Check sheet for the modelled part. Datum: model origin and axes. Units: mm. A direction names the side the tool comes from. Give positions to 0.01 mm unless a question says otherwise; leave off trailing zeros. Write each loop counter-clockwise with the first axis right and the second up, starting at its lowest first coordinate (ties: lowest second). Pieces come first, ordered by that corner, then holes. Notation, with made-up numbers: (-25.75, -9) -> (31.25, -9) arc R15 cw to (31.25, 7) -> close; hole circle Ø3 at (40.5, 18.25). An arc over 180 degrees is marked (long way). Use a Markdown table: item, result. Add a question column.
1. Cross-section at B-B (z = -26.7). Enter the section's corners in (x, y).
2. Scan lines: probe 1 along X at (y, z) = (2.5, 40.5); probe 2 along X at (y, z) = (3.8, 16.25); probe 3 along Z at (x, y) = (-18, 7). Record each from-to range of solid material in increasing order. Write a range as [from, to].
3. Cross-section at C-C (z = 0). Enter the section's corners in (x, y), then the cut area to 3 significant figures.
4. Set-up check for faces 1 (the flat face through (-49.65, 5, -7)), 2 (the flat face through (10.75, 4, -39)), 3 (the flat face through (18, 5, 1)): record each of +Z, -Z, +X, -X, +Y, -Y from which the full face is reachable in a straight line by a thin tool's end or side.
5. Cross-section at A-A (x = -36.95). Enter the section's corners in (y, z), then the cut area to 3 significant figures.
6. Release check for a two-part mould opening along X. For faces 4 (the flat face through (-12.75, 3, 1)), 5 (the flat face through (-21.25, 7, 1)), 6 (the flat face through (-51, 7, 10)) record: released by +X, released by -X, zero draft, split by the parting line, or undercut.
7. Cross-section at D-D (x = 0). Count the separate pieces of the cut face and the enclosed holes in it, then the cut area to 3 significant figures.
8. Gauge pin test, flat ends, axial feed: P1, Ø4, axis at x = -14.5, z = 10.5, coming from the +Y side; P2, Ø4, axis at y = 8, z = 13, coming from the -X side; P3, Ø1.5, axis at x = -27, y = 7.5, coming from the -Z side. Record the tip position at first contact, or that the pin passes through.
from build123d import *

# Parameters (mm, degrees)
BOSS_EXTRUDE1_DEPTH            = 45
SKETCH3_R                      = 6.5
CUT_EXTRUDE1_DEPTH             = 50.199212392
SKETCH5_W                      = 5
SKETCH5_H                      = 10
BOSS_EXTRUDE2_DEPTH            = 45
BOSS_EXTRUDE2_DEPTH_BACK       = 45
SKETCH8_W                      = 43.5
SKETCH8_H                      = 10
BOSS_EXTRUDE3_DEPTH            = 3
MOVE_FACE1_BY                  = 1
MOVE_FACE2_BY                  = 1
SKETCH10_W                     = 6.1
SKETCH10_H                     = 1.6
CUT_EXTRUDE2_DEPTH             = 3.5
CBORE_FOR_M2_SHCS1_D           = 2.4
CBORE_FOR_M2_SHCS1_CBORE_D     = 4.4
CBORE_FOR_M2_SHCS1_CBORE_DEPTH = 3
SKETCH12_W                     = 10
SKETCH12_H                     = 10
BOSS_EXTRUDE4_DEPTH            = 25.4
SKETCH13_W                     = 3
SKETCH13_H                     = 10
BOSS_EXTRUDE5_DEPTH            = 10
FILLET1_R                      = 3
CHAMFER1_SIZE                  = 5
FILLET2_R                      = 1
MOVE_FACE3_BY                  = 2
M2_CLEARANCE_HOLE1_D           = 2.4
SKETCH18_W                     = 21.5
SKETCH18_H                     = 23.75
SKETCH18_H_2                   = 11.7
SKETCH18_H_3                   = 13.3
CUT_EXTRUDE4_DEPTH             = 2
FILLET4_R                      = 1


with BuildPart() as part:
    # Sketch2 → Boss-Extrude1 (new, symmetric)
    with BuildSketch(Plane.XY):
        Polygon((-19.25, 0), (19.25, 0), (19.25, 5), (16.25, 5), (16.25, 1.9), (12.75, 1.9), (12.75, 5), (-12.75, 5), (-12.75, 1.9), (-16.25, 1.9), (-16.25, 5), (-19.25, 5), align=None)
    extrude(amount=BOSS_EXTRUDE1_DEPTH, both=True)

    # Sketch3 → Cut-Extrude1 (cut, through all)
    with BuildSketch(Plane.XZ):
        with Locations(Location((0, 0, 0), (0, 0, 270))):
            Circle(SKETCH3_R)
    extrude(amount=-CUT_EXTRUDE1_DEPTH, mode=Mode.SUBTRACT)

    # Sketch5 → Boss-Extrude2 (add, two sides)
    with BuildSketch(Plane.XY) as boss_extrude2_sk:
        with Locations((-21.75, 5)):
            Rectangle(SKETCH5_W, SKETCH5_H)
    extrude(amount=BOSS_EXTRUDE2_DEPTH)
    extrude(boss_extrude2_sk.sketch, amount=-BOSS_EXTRUDE2_DEPTH_BACK)

    # Sketch8 → Boss-Extrude3 (add)
    with BuildSketch(Plane.XY.offset(45)):
        with Locations((-2.5, 5)):
            Rectangle(SKETCH8_W, SKETCH8_H)
    boss_extrude3 = extrude(amount=BOSS_EXTRUDE3_DEPTH)

    # Mirror1: Boss-Extrude3 across plane
    add(boss_extrude3.mirror(Plane.XY))

    # Move Face1: a face moved outward by 1.0
    extrude(part.faces().sort_by_distance((-2.5, 5, -48))[0], amount=MOVE_FACE1_BY, dir=(0, 0, -1))

    # Move Face2: a face moved outward by 1.0
    extrude(part.faces().sort_by_distance((-2.5, 5, 48))[0], amount=MOVE_FACE2_BY, dir=(0, 0, 1))

    # Sketch10 → Cut-Extrude2 (cut)
    with BuildSketch(Plane(origin=(0, 10, 0), x_dir=(1, 0, 0), z_dir=(0, 1, 0))):
        with Locations((-16.3, 47)):
            Rectangle(SKETCH10_W, SKETCH10_H)
        with Locations((11.3, 47)):
            Rectangle(SKETCH10_W, SKETCH10_H)
        with Locations((-16.3, -47)):
            Rectangle(SKETCH10_W, SKETCH10_H)
        with Locations((11.3, -47)):
            Rectangle(SKETCH10_W, SKETCH10_H)
    extrude(amount=-CUT_EXTRUDE2_DEPTH, mode=Mode.SUBTRACT)

    # CBORE for M2 SHCS1 (through all)
    with Locations(Plane(origin=(0, 5, 0), x_dir=(1, 0, 0), z_dir=(0, 1, 0))):
        with Locations((0, 26.7), (0, -16.25)):
            CounterBoreHole(CBORE_FOR_M2_SHCS1_D / 2, CBORE_FOR_M2_SHCS1_CBORE_D / 2, CBORE_FOR_M2_SHCS1_CBORE_DEPTH)

    # Sketch12 → Boss-Extrude4 (add)
    with BuildSketch(Plane.ZY.offset(24.25)):
        with Locations((0, 5)):
            Rectangle(SKETCH12_W, SKETCH12_H)
    extrude(amount=BOSS_EXTRUDE4_DEPTH)

    # Sketch13 → Boss-Extrude5 (add, symmetric)
    with BuildSketch(Plane.XY):
        with Locations((-51.15, 5)):
            Rectangle(SKETCH13_W, SKETCH13_H)
    extrude(amount=BOSS_EXTRUDE5_DEPTH, both=True)

    # Fillet1
    fillet1_edges = [part.edges().sort_by_distance(p)[0] for p in [
        (-51.15, 0, -10),
        (-51.15, 0, 10),
    ]]
    fillet(fillet1_edges, radius=FILLET1_R)

    # Chamfer1
    chamfer1_edges = [part.edges().sort_by_distance(p)[0] for p in [
        (-2.5, 0, 49),
        (-2.5, 0, -49),
    ]]
    chamfer(chamfer1_edges, length=CHAMFER1_SIZE)

    # Fillet2
    fillet2_edges = [part.edges().sort_by_distance(p)[0] for p in [
        (-2.5, 0, 44),
        (-2.5, 0, -44),
        (-2.5, 5, -49),
        (-2.5, 5, 49),
    ]]
    fillet(fillet2_edges, radius=FILLET2_R)

    # Move Face3: a face moved inward by 2.0
    extrude(part.faces().sort_by_distance((-19.25, 7.5, 0))[0], amount=MOVE_FACE3_BY, dir=(-1, 0, 0), mode=Mode.SUBTRACT)

    # M2 Clearance Hole1 (through all)
    with Locations(Plane(origin=(0, 10, 0), x_dir=(1, 0, 0), z_dir=(0, 1, 0))):
        with Locations((-36.95, 0)):
            Hole(M2_CLEARANCE_HOLE1_D / 2)

    # Sketch18 → Cut-Extrude4 (cut)
    with BuildSketch(Plane(origin=(0, 5, 0), x_dir=(1, 0, 0), z_dir=(0, 1, 0))):
        with Locations((0, -33.125)):
            Rectangle(SKETCH18_W, SKETCH18_H)
        with Locations((0, 15.85)):
            Rectangle(SKETCH18_W, SKETCH18_H_2)
        with Locations((0, 38.35)):
            Rectangle(SKETCH18_W, SKETCH18_H_3)
    extrude(amount=-CUT_EXTRUDE4_DEPTH, mode=Mode.SUBTRACT)

    # Fillet4
    fillet4_edges = [part.edges().sort_by_distance(p)[0] for p in [
        (-10.75, 4, 21.25),
        (10.75, 4, 21.25),
        (-10.75, 4, -10),
        (-10.75, 4, -21.7),
        (10.75, 4, -21.7),
        (10.75, 4, -10),
        (-10.75, 4, -31.7),
        (10.75, 4, -31.7),
    ]]
    fillet(fillet4_edges, radius=FILLET4_R)


solid = part.part
Worked answers:
| question | item | result |
|---|---|---|
| 1 | outline | (-24.25, 0) -> (-1.2, 0) -> (-1.2, 2) -> (-2.2, 2) -> (-2.2, 5) -> (-12.75, 5) -> (-12.75, 1.9) -> (-16.25, 1.9) -> (-16.25, 5) -> (-21.25, 5) -> (-21.25, 10) -> (-24.25, 10) -> close; (1.2, 0) -> (19.25, 0) -> (19.25, 5) -> (16.25, 5) -> (16.25, 1.9) -> (12.75, 1.9) -> (12.75, 5) -> (2.2, 5) -> (2.2, 2) -> (1.2, 2) -> close |
| 2 | probe 1 | x = [-24.25, -16.25], [-12.75, 12.75], [16.25, 19.25] |
| 2 | probe 2 | x = [-24.25, -16.25], [-12.75, -2.2], [2.2, 12.75], [16.25, 19.25] |
| 2 | probe 3 | z = [-49, -47.8], [-46.2, -45], [45, 46.2], [47.8, 49] |
| 3 | outline | (-52.65, 0) -> (-38.15, 0) -> (-38.15, 10) -> (-52.65, 10) -> close; (-35.75, 0) -> (-6.5, 0) -> (-6.5, 5) -> (-12.75, 5) -> (-12.75, 1.9) -> (-16.25, 1.9) -> (-16.25, 5) -> (-21.25, 5) -> (-21.25, 10) -> (-35.75, 10) -> close; (6.5, 0) -> (19.25, 0) -> (19.25, 5) -> (16.25, 5) -> (16.25, 1.9) -> (12.75, 1.9) -> (12.75, 5) -> (6.5, 5) -> close |
| 3 | area | 406 mm² |
| 4 | face 1 | -Z, +Y, -Y |
| 4 | face 2 | +Y |
| 4 | face 3 | +X, +Y |
| 5 | outline | (0, -5) -> (10, -5) -> (10, -1.2) -> (0, -1.2) -> close; (0, 1.2) -> (10, 1.2) -> (10, 5) -> (0, 5) -> close |
| 5 | area | 76.0 mm² |
| 6 | face 4 | undercut |
| 6 | face 5 | released by +X |
| 6 | face 6 | zero draft |
| 7 | separate pieces | 4 |
| 7 | enclosed holes | 0 |
| 7 | area | 306 mm² |
| 8 | P1 | stops at y = 5 |
| 8 | P2 | stops at x = -24.25 |
| 8 | P3 | stops at z = -5 |
